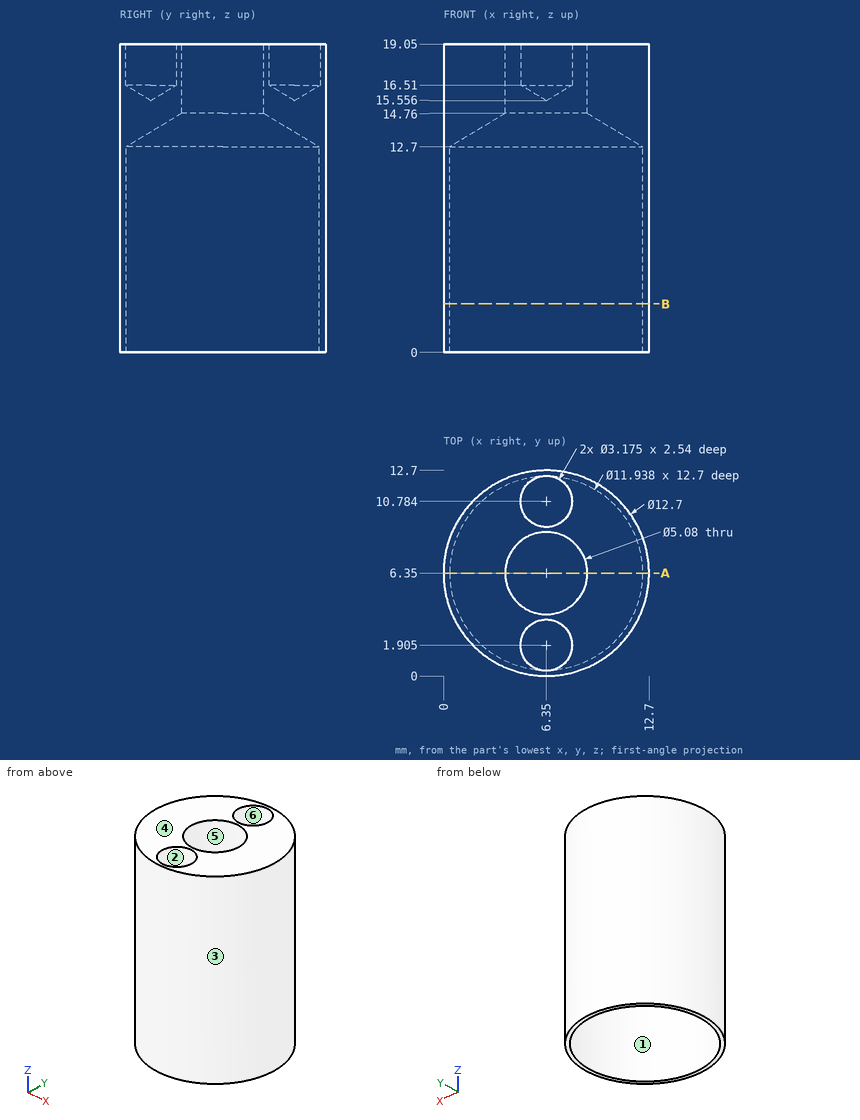
Here's the drawing with two shaded views (mm, measured from the low corner). I have some questions. A direction names the side the tool comes from. Give positions to 0.01 mm unless a question says otherwise; leave off trailing zeros. Loops run counter-clockwise (first coordinate to the right, second up) from the corner with the lowest first, then second, coordinate; pieces in that order, holes last. Notation, with made-up numbers: (36, 31) -> (95, 31) arc R17 ccw to (95, 57) -> close; hole circle Ø10 at (-19, 26). An arc over 180 degrees is marked (long way). One line per item, written item: value.
Q1. Suppose I cut it at A-A on y = 6.35. Please give me the cut outline in (x, z).
Answers follow:
outline: (0, 0) -> (0.38, 0) -> (0.38, 12.7) -> (3.81, 14.76) -> (3.81, 19.05) -> (0, 19.05) -> close; (8.89, 14.76) -> (12.32, 12.7) -> (12.32, 0) -> (12.7, 0) -> (12.7, 19.05) -> (8.89, 19.05) -> close
Q2. On a 3-axis mill with a long thin cutter (end or side, diameter ignored), from which of +Z, -Z, +X, -X, +Y, -Y can I reach the whole of each face in a straight line? I mean the marked faces 1 and 2. Say none if no direction works.
Answers follow:
face 1: -Z
face 2: +Z
Q3. If I drill on line 1 along Y through (x, z) = (6.35, 18.45); line 2 along Y through (x, z) = (9, 6.5); line 3 along Y through (x, z) = (4.5, 17.75) (1 decimal), over which ranges is the centre line in solid material (lowest first)?
Answers follow:
line 1: 0 to 0.32, 3.49 to 3.81, 8.89 to 9.2, 12.37 to 12.7
line 2: 0.58 to 1, 11.7 to 12.12
line 3: 0.3 to 4.6, 8.1 to 12.4
Q4. We'd pull the mould along X, two halves only. Please class the marked faces 3, 4, 5 and 6: pulls with the +X half, pulls with the -X half, needs draft (parallel to the pull), parting line crosses it, or undercut.
Answers follow:
face 3: parting line crosses it
face 4: needs draft
face 5: undercut
face 6: undercut
Q5. I'm going to push flat-ended pins straight in: pin 1 Ø1.5 at (y, z) = (9.5, 13) entering from +X; pin 2 Ø2 at (x, y) = (10.5, 7.5) entering from -Z; pin 3 Ø5 at (y, z) = (1.5, 5.5) entering from -X; pin 4 Ø4 at (x, y) = (6.35, 6.35) entering from -Z. Where does each tip first touch, or does it pass through?
Answers follow:
pin 1: x = 12.23
pin 2: z = 13.1
pin 3: x = 0.45
pin 4: through
Q6. Suppose I cut it at B-B on z = 3. Please give me the cut outline in (x, y).
Answers follow:
outline: circle Ø12.7 at (6.35, 6.35); hole circle Ø11.94 at (6.35, 6.35)
